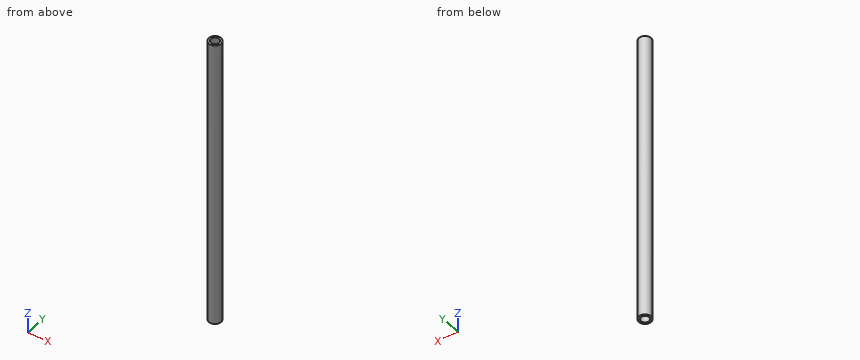
Autodesk Inventor part; units mm, degrees
ref_plane "YZ Plane" through (0, 0, 0) normal (1, 0, 0) x (0, 1, 0)
ref_plane "XZ Plane" through (0, 0, 0) normal (0, 1, 0) x (-1, 0, 0)
ref_plane "XY Plane" through (0, 0, 0) normal (0, 0, 1) x (1, 0, 0)
sketch "Sketch1" plane through (0, 0, 0) normal (0, 0, 1) x (1, 0, 0)
  circle A0 centre (0, 0) radius 1.5875
  dimension "d0" = 3.175
extrude "Extrusion1" add sketch "Sketch1" along normal blind 76.2
sketch "Sketch2" plane through (0, 0, 76.2) normal (0, 0, 1) x (1, 0, 0)
  circle A0 centre (0, 0) radius 1.5875
  circle A1 centre (0, 0) radius 1.1303
  dimension "d3" = 2.2606
hole "Hole1" at (0, 0, 76.2) direction (0, 0, -1) diameter 2.159 depth 25.4 tip angle 118
sketch "Sketch3" plane through (0, 0, 0) normal (0, 0, -1) x (-1, 0, 0)
  circle A0 centre (0, 0) radius 1.5875
hole "Hole2" at (0, 0, 0) direction (0, 0, 1) diameter 2.159 depth 25.4 tip angle 118
properties part number "Steel Rod"
The listing builds one solid part. Answer for the finished solid, in the listing's coordinates (mm). Coordinates: 2 decimals unless noted, no trailing zeros. Order: outer loops, then holes, each group sorted by start corner. A loop starts at its lowest first (then second) coordinate and runs counter-clockwise, first axis right, second up. Notation, with made-up numbers: M 80,-9.5 L 108,-9.5 A7 ccw 108,1.5 Z; hole C 86,0 d5. An arc over 180 degrees is marked long. Answer as a JSON object with one key per item and string values. Group by question number.
1. Flat-ended cylindrical pins translate along their axes: P1, Ø1.5, axis at y = 1, z = 67, coming from the -X side; P2, Ø1.7, axis at x = 0, y = 0, coming from the -Z side. Find the tip coordinate at first contact, or state that the pin passes through.
2. Section B-B on z = 59.5 is taken. Write down the section's boundary in (x, y) (1 decimal), then the cut area to 3 significant figures.
3. Section A-A on z = 27 is taken. Write down the section's boundary in (x, y) (1 decimal), then the cut area to 3 significant figures.
4. Straight lines are drawn through the part: line 1 (Y direction, x = 0.15, z = 65); line 2 (X direction, y = 0.1, z = 39); line 3 (X direction, y = -0.35, z = 64). For each, find the intervals that lie inside material, in ascending order.
Values follow:
{
 "1": {"P1": "x = -1.57", "P2": "z = 25.54"},
 "2": {"outline": "C 0,0 d3.2; hole C 0,0 d2.2", "area": "4.26 mm2"},
 "3": {"outline": "C 0,0 d3.2", "area": "7.92 mm2"},
 "4": {"line 1": "-1.58 to -1.07, 1.07 to 1.58", "line 2": "-1.58 to 1.58", "line 3": "-1.55 to -1.02, 1.02 to 1.55"}
}
